```python
from build123d import *

# Parameters (mm, degrees)
SKETCH1_W           = 410
SKETCH1_H           = 150
BOSS_EXTRUDE1_DEPTH = 35
SKETCH2_W           = 410
SKETCH2_H           = 5
BOSS_EXTRUDE2_DEPTH = 150
SKETCH3_W           = 80
SKETCH3_H           = 150
CUT_EXTRUDE1_DEPTH  = 30
SKETCH4_W           = 210
SKETCH4_H           = 145
CUT_EXTRUDE2_DEPTH  = 35
SKETCH5_W           = 120
SKETCH5_H           = 120
CUT_EXTRUDE3_DEPTH  = 10
SKETCH6_W           = 50
SKETCH6_H           = 120
CUT_EXTRUDE4_DEPTH  = 10


with BuildPart() as part:
    # Sketch1 → Boss-Extrude1 (new body)
    with BuildSketch(Plane.XY):
        with Locations((205, 75)):
            Rectangle(SKETCH1_W, SKETCH1_H)
    extrude(amount=BOSS_EXTRUDE1_DEPTH)

    # Sketch2 → Boss-Extrude2 (add)
    with BuildSketch(Plane(origin=(0, 0, 0), x_dir=(-1, 0, 0), z_dir=(0, 0, -1))):
        with Locations((-205, 147.5)):
            Rectangle(SKETCH2_W, SKETCH2_H)
    extrude(amount=BOSS_EXTRUDE2_DEPTH)

    # Sketch3 → Cut-Extrude1 (cut)
    with BuildSketch(Plane.XY.offset(35)):
        with Locations((50, 75)):
            Rectangle(SKETCH3_W, SKETCH3_H)
        with Locations((360, 75)):
            Rectangle(SKETCH3_W, SKETCH3_H)
    extrude(amount=-CUT_EXTRUDE1_DEPTH, mode=Mode.SUBTRACT)

    # Sketch4 → Cut-Extrude2 (cut)
    with BuildSketch(Plane.XY.offset(35)):
        with Locations((205, 72.5)):
            Rectangle(SKETCH4_W, SKETCH4_H)
    extrude(amount=-CUT_EXTRUDE2_DEPTH, mode=Mode.SUBTRACT)

    # Sketch5 → Cut-Extrude3 (cut)
    with BuildSketch(Plane(origin=(0, 150, 0), x_dir=(1, 0, 0), z_dir=(0, 1, 0))):
        with Locations((60, 90)):
            Rectangle(SKETCH5_W, SKETCH5_H)
    extrude(amount=-CUT_EXTRUDE3_DEPTH, mode=Mode.SUBTRACT)

    # Sketch6 → Cut-Extrude4 (cut)
    with BuildSketch(Plane(origin=(0, 150, 0), x_dir=(1, 0, 0), z_dir=(0, 1, 0))):
        with Locations((385, 90)):
            Rectangle(SKETCH6_W, SKETCH6_H)
    extrude(amount=-CUT_EXTRUDE4_DEPTH, mode=Mode.SUBTRACT)


solid = part.part
```
Verification items for the finished model (mm, model axes). A direction names the side the tool comes from. Coordinates: 2 decimals unless noted, no trailing zeros. Order: outer loops, then holes, each group sorted by start corner. A loop starts at its lowest first (then second) coordinate and runs counter-clockwise, first axis right, second up. Notation, with made-up numbers: (18.25, -29) -> (42.25, -29) arc R17 ccw to (42.25, -3) -> close; hole circle Ø2 at (72.25, 7.25). An arc over 180 degrees is marked (long way). Answer as CSV lines item,"result". Start each with the question number.
1) Cross-section at A-A, the plane y = 100. Record the boundary of the cut face in (x, z).
2) Release check for a two-part mould opening along X. For faces 1 (the face through (253, 145, -56)), 2 (the face through (204, 148, 35)), 3 (the face through (0, 74, 17)), 4 (the face through (320, 74, 20)) record: released by +X, released by -X, zero draft, split by the parting line, or undercut.
3) Material ranges on L1, parallel to X at y = 7, z = 22; L2, parallel to Z at x = 346, y = 21.5; L3, parallel to Y at x = 265, z = -4, recorded low to high. Write a range as [from, to].
4) Cross-section at B-B, the plane z = 12.5. Record the boundary of the cut face in (x, y).
5) Gauge pin test, flat ends, axial feed: pin 1 Ø4 at (x, y) = (53.5, 148.5) entering from -Z; pin 2 Ø12 at (x, y) = (81.5, 49.5) entering from +Z; pin 3 Ø10 at (x, z) = (102, -30.5) entering from -Y. Record the tip position at first contact, or that the pin passes through.
6) Set-up check for faces 5 (the face through (400, 74, 20)), 6 (the face through (310, 71, 18)), 7 (the face through (359, 74, 0)): record each of +Z, -Z, +X, -X, +Y, -Y from which the full face is reachable in a straight line by a thin tool's end or side.
7) Cross-section at D-D, the plane z = -57. Record the boundary of the cut face in (x, y).
8) Cross-section at C-C, the plane x = 52.5. Record the boundary of the cut face in (y, z), then the cut area to 3 significant figures.
Conclusion:
1,outline,"(0, 0) -> (100, 0) -> (100, 35) -> (90, 35) -> (90, 5) -> (10, 5) -> (10, 35) -> (0, 35) -> close; (310, 0) -> (410, 0) -> (410, 35) -> (400, 35) -> (400, 5) -> (320, 5) -> (320, 35) -> (310, 35) -> close"
2,face 1,"undercut"
2,face 2,"zero draft"
2,face 3,"released by -X"
2,face 4,"undercut"
3,L1,"x = [0, 10], [90, 100], [310, 320], [400, 410]"
3,L2,"z = [0, 5]"
3,L3,"y = [145, 150]"
4,outline,"(0, 0) -> (10, 0) -> (10, 150) -> (0, 150) -> close; (90, 0) -> (100, 0) -> (100, 145) -> (310, 145) -> (310, 0) -> (320, 0) -> (320, 150) -> (90, 150) -> close; (400, 0) -> (410, 0) -> (410, 150) -> (400, 150) -> close"
5,pin 1,"stops at z = -30"
5,pin 2,"stops at z = 5"
5,pin 3,"stops at y = 145"
6,face 5,"+Z, +Y, -Y"
6,face 6,"+Z, -Z, -Y"
6,face 7,"-Z, +X, -X, -Y"
7,outline,"(120, 145) -> (360, 145) -> (360, 150) -> (120, 150) -> close"
8,outline,"(0, 0) -> (145, 0) -> (145, -30) -> (150, -30) -> (150, 5) -> (0, 5) -> close"
8,area,"900 mm²"
